Design review of the part built by this model. Coordinates are the model's own, in mm. Coordinates: 2 decimals unless noted, no trailing zeros. Use a Markdown table: item, result. Add a question column.
Q1. Draft analysis for pull direction X (two halves, no side actions). For faces 1 (the face through (1.17, 5.27, -14.65)), 2 (the face through (0, -6, -40)), 3 (the face through (11.99, 0.53, -30.95)), state which applies: pulls with the +X half, pulls with the -X half, needs draft (parallel to the pull), parting line crosses it, or undercut.
Q2. Clearance check with flat-ended pins moving along their axes: pin 1 Ø5 at (y, z) = (8.5, -8.5) entering from +X; pin 2 Ø6 at (y, z) = (18.5, 2.5) entering from +X; pin 3 Ø8 at (y, z) = (14, -13) entering from -X. State where each tip first meets the part, or that it passes through.
Q3. For probe 1 along Y at (x, z) = (0, -28); probe 2 along Y at (x, z) = (0, -21); probe 3 along Z at (x, y) = (10, -18), list the stretches that pass through material, from the lowest coordinate up.
from build123d import *

# Parameters (mm, degrees)
F3_D           = 10.8
F3_DEPTH       = 50
F3_CBORE_D     = 10.8
F3_CBORE_DEPTH = 10.8
F3_TIP         = 3.2446473427


with BuildPart() as f1:
    # F0 (on Front) → F1 (revolve)
    with BuildSketch(Plane.XZ):
        with BuildLine():
            Line((0, -40), (0, 25))
            add(Edge.make_bspline(
                [(0, 25), (-78.1095262892, 25), (-14.5161290323, -20.3539184905)],
                knots=[4.7123889804, 4.7123889804, 4.7123889804, 7.2344607382, 7.2344607382, 7.2344607382], degree=2, weights=[1, 0.3048304942, 1]))
            ThreePointArc((-14.5161290323, -20.3539184905), (-12.665994666, -22.4914261089), (-12, -25.2388589282))
            Line((-12, -25.2388589282), (-12, -36.5))
            ThreePointArc((-12, -36.5), (-10.9748737342, -38.9748737342), (-8.5, -40))
            Line((-8.5, -40), (0, -40))
        make_face()
    revolve(axis=Axis((0, 0, -7.5), (0, 0, -1)))

    # F3
    with Locations(Plane(origin=(0, 0, -40), x_dir=(1, 0, 0), z_dir=(0, 0, -1))):
        with Locations((0, 0)):
            CounterBoreHole(F3_D / 2, F3_CBORE_D / 2, F3_CBORE_DEPTH, depth=F3_DEPTH)
            with Locations((0, 0, -(F3_DEPTH + F3_TIP / 2))):  # 118° drill point
                Cone(0, F3_D / 2, F3_TIP, mode=Mode.SUBTRACT)


solid = f1.part
Answer list:
| question | item | result |
|---|---|---|
| 1 | face 1 | undercut |
| 1 | face 2 | needs draft |
| 1 | face 3 | parting line crosses it |
| 2 | pin 1 | x = 23.12 |
| 2 | pin 2 | x = 19.48 |
| 2 | pin 3 | x = -19.92 |
| 3 | probe 1 | -12 to -5.4, 5.4 to 12 |
| 3 | probe 2 | -13.75 to -5.4, 5.4 to 13.75 |
| 3 | probe 3 | -14.18 to 14.18 |
